Geometry check sheet. Reference: the model listing, model coordinates, mm. Coordinates: 2 decimals unless noted, no trailing zeros. Write each loop counter-clockwise with the first axis right and the second up, starting at its lowest first coordinate (ties: lowest second). Pieces come first, ordered by that corner, then holes. Notation, with made-up numbers: M -6.5,28.25 L 40.5,28.25 A5 ccw 40.5,32.25 Z; hole C 17.25,2.25 d9. An arc over 180 degrees is marked long. Write each question's results on one line, items separated by ' | '.
Autodesk Inventor part; units mm, degrees
ref_plane "YZ Plane" through (0, 0, 0) normal (1, 0, 0) x (0, 1, 0)
ref_plane "XZ Plane" through (0, 0, 0) normal (0, 1, 0) x (-1, 0, 0)
ref_plane "XY Plane" through (0, 0, 0) normal (0, 0, 1) x (1, 0, 0)
sketch "Sketch1" plane through (0, 0, 0) normal (0, 0, 1) x (1, 0, 0)
  circle A0 centre (0, 0) radius 1.5
  dimension "d0" = 3
extrude "Extrusion1" add sketch "Sketch1" along normal blind 8
fillet "Fillet1" radius 0.1 1 edges at (-1.5, 0, 8)
sketch "Sketch2" plane through (0, 0, 0) normal (0, 0, -1) x (-1, 0, 0)
  circle A0 centre (0, 0) radius 2.5
  dimension "d4" = 5
extrude "Extrusion2" add sketch "Sketch2" along normal blind 1
sketch "Sketch3" plane through (0, 0, -1) normal (0, 0, -1) x (-1, 0, 0)
  line L0 (-1.4142, 0.5) -> (1.4142, 0.5)
  line L1 (1.4142, 0.5) -> (1.4142, -0.5)
  line L2 (1.4142, -0.5) -> (-1.4142, -0.5)
  line L3 (-1.4142, -0.5) -> (-1.4142, 0.5)
  line L4 (-1.4142, 0.5) -> (1.4142, -0.5) construction
  line L5 (1.4142, 0.5) -> (-1.4142, -0.5) construction
  line L6 (0.5, 1.4142) -> (-0.5, 1.4142)
  line L7 (-0.5, 1.4142) -> (-0.5, -1.4142)
  line L8 (-0.5, -1.4142) -> (0.5, -1.4142)
  line L9 (0.5, -1.4142) -> (0.5, 1.4142)
  line L10 (0.5, 1.4142) -> (-0.5, -1.4142) construction
  line L11 (-0.5, 1.4142) -> (0.5, -1.4142) construction
  point P0 (0, 0)
  point P1 (0, 0)
  point P2 (0, 0)
  dimension "d8" = 1
  dimension "d9" = 1
extrude "Extrusion3" cut sketch "Sketch3" against normal blind 0.5
fillet "Fillet2" radius 0.6 1 edges at (2.5, 0, -1)
properties part number "M3"
Q1. Mould release check, pull along Y, two halves, no side actions. Record for faces 1 (the flat face through (0, 0, -0.5)), 2 (the cylindrical face through (-1.5, -0.07, 3.89)), 3 (the flat face through (-2, 0, 0)): pulls with the +Y half, pulls with the -Y half, needs draft (parallel to the pull), parting line crosses it, or undercut.
Geometry check:
face 1: undercut | face 2: parting line crosses it | face 3: needs draft
Q2. Scan lines: probe 1 along Z at (x, y) = (0.2, 0.3); probe 2 along Z at (x, y) = (-1.85, 0.6); probe 3 along Y at (x, z) = (-0.5, 3). Record each from-to range of solid material in increasing order.
Geometry check:
probe 1: z = -0.5 to 8 | probe 2: z = -1 to 0 | probe 3: y = -1.41 to 1.41
Q3. Sectioned sample at C-C on z = 0.75. Record the cut outline in (x, y), and give its area (3 significant figures).
Geometry check:
outline: C 0,0 d3 | area: 7.07 mm2
Q4. Depth check by flat-ended pin: P1, Ø1.5, axis at y = 0.5, z = 4, coming from the +X side; P2, Ø2.5, axis at x = 0, y = 0.5, coming from the -Z side; P3, Ø3, axis at y = 0, z = 3.5, coming from the -X side. Enter the tip coordinate at first touch or a pass-through.
Geometry check:
P1: stops at x = 1.5 | P2: stops at z = -1 | P3: stops at x = -1.5
Q5. Sectioned sample at A-A on x = 0. Record the cut outline in (y, z), and give its area (3 significant figures).
Geometry check:
outline: M -2.5,-0.4 A0.6 ccw -1.9,-1 L -1.41,-1 L -1.41,-0.5 L 1.41,-0.5 L 1.41,-1 L 1.9,-1 A0.6 ccw 2.5,-0.4 L 2.5,0 L 1.5,0 L 1.5,7.9 A0.1 ccw 1.4,8 L -1.4,8 A0.1 ccw -1.5,7.9 L -1.5,0 L -2.5,0 Z | area: 27.4 mm2
